Autodesk Fusion 360 part; units mm, degrees
sketch "Sketch2" plane through (0, 0, 0) normal (0, 0, 1) x (1, 0, 0)
  line L0 (0, 0) -> (0, 6)
  line L1 (4, 6) -> (4, 0)
  line L2 (4, 0) -> (0, 0)
  line L3 (1, 6) -> (2, 5)
  line L4 (2, 5) -> (3, 6)
  line L5 (0, 6) -> (1, 6)
  line L6 (3, 6) -> (4, 6)
  dimension "d12" = 4
  dimension "d13" = 1
  dimension "d14" = 1
  dimension "d15" = 6
revolve "Revolve1" add sketch "Sketch2" angle 360 about axis through (4, 0, 0) along (-1, 0, 0)
sketch "Sketch3" plane through (4, 0, 0) normal (1, 0, 0) x (0, 1, 0)
  circle A0 centre (0, 0) radius 6
  circle A1 centre (0, 0) radius 1.5
  dimension "d18" = 3
extrude "Extrude2" cut sketch "Sketch3" against normal through all contours A1
sketch "Sketch4" plane through (4, 0, 0) normal (1, 0, 0) x (0, 1, 0)
  circle A0 centre (0, 0) radius 1.5
  circle A1 centre (0, 0) radius 6
  circle A2 centre (0, 0) radius 3.5
  circle A3 centre (0, 0) radius 2
  dimension "d20" = 7
  dimension "d21" = 4
extrude "Extrude3" cut sketch "Sketch4" against normal blind 0.1 contours A2
sketch "Sketch5" plane through (0, 0, 0) normal (-1, 0, 0) x (0, -1, 0)
  circle A0 centre (0, 0) radius 1.5
  circle A1 centre (0, 0) radius 6
  circle A2 centre (0, 0) radius 2
  circle A3 centre (0, 0) radius 3.5
  dimension "d24" = 7
  dimension "d25" = 4
extrude "Extrude4" cut sketch "Sketch5" against normal blind 0.1 contours A3
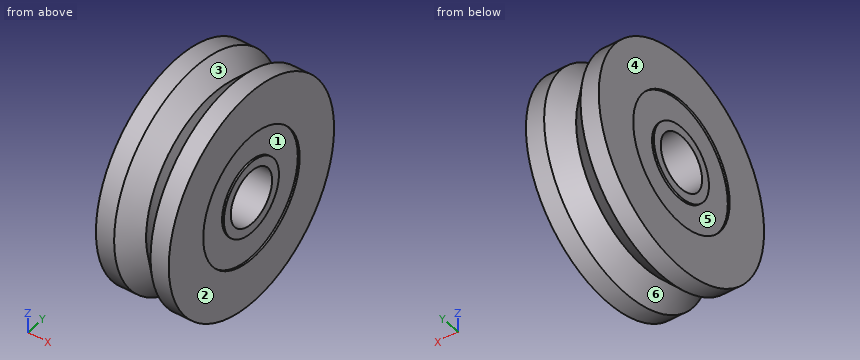
Work out the finished part from the listing and answer in its coordinate system (mm). Face numbers are marked on the shaded views. A direction names the side the tool comes from. Coordinates: 2 decimals unless noted, no trailing zeros. Loops run counter-clockwise (first coordinate to the right, second up) from the corner with the lowest first, then second, coordinate; pieces in that order, holes last. Notation, with made-up numbers: M -2.75,9.25 L 44.25,9.25 A27 cw 44.25,36.25 Z; hole C 2.25,38 d3. An arc over 180 degrees is marked long. Answer in a Markdown table with one row per item. Add a question column.
1. Consider L1, parallel to Z at x = 3.95, y = 0; L2, parallel to X at y = -5.5, z = -1; L3, parallel to Z at x = 2.7, y = -0.75. Determine where each line is inside the solid, lowest interval first.
2. A tool of negligible diameter and unlimited length cuts with its end or side. For the marked faces 4, 5 and 6, from which of +Z, -Z, +X, -X, +Y, -Y can it reach the whole face along a straight path? Write none if from no direction.
3. Find section C-C, the plane x = 0.45. Write down the section's boundary in (y, z).
4. The mould has two halves that part along Y. Classify the marked faces 1, 2 and 3: pulls with the +Y half, pulls with the -Y half, needs draft (parallel to the pull), parting line crosses it, or undercut.
5. A flat-ended cylindrical pin translates along its axis: P1, Ø1.8, axis at y = 0, z = 0, coming from the +X side. Find the tip coordinate at first contact, or state that the pin passes through.
6. Find section D-D, the plane x = 2.5. Write down the section's boundary in (y, z), then the cut area to 3 significant figures.
Reported:
| question | item | result |
|---|---|---|
| 1 | L1 | z = -6 to -3.5, -2 to -1.5, 1.5 to 2, 3.5 to 6 |
| 1 | L2 | x = 0 to 1.41, 2.59 to 4 |
| 1 | L3 | z = -5.65 to -1.3, 1.3 to 5.65 |
| 2 | face 4 | +Z, -Z, -X, +Y, -Y |
| 2 | face 5 | -X |
| 2 | face 6 | none |
| 3 | outline | C 0,0 d12; hole C 0,0 d3 |
| 4 | face 1 | undercut |
| 4 | face 2 | needs draft |
| 4 | face 3 | parting line crosses it |
| 5 | P1 | passes through |
| 6 | outline | C 0,0 d11; hole C 0,0 d3 |
| 6 | area | 88.0 mm^2 |
